Drawing for the job (mm, zero at the part's lowest x, y, z). Round coordinates to 2 decimals unless told otherwise and drop trailing zeros. Loops run counter-clockwise (first coordinate to the right, second up) from the corner with the lowest first, then second, coordinate; pieces in that order, holes last. Notation, with made-up numbers: (18.5, 84.25) -> (74.5, 84.25) arc R25 ccw to (74.5, 114.25) -> close; hole circle Ø11 at (32.25, 47). An arc over 180 degrees is marked (long way). Put each result on its own line as item: value. Start each with the question number.
Item 1: Cut at B-B, the plane x = 20. List the corners of the cut face in (y, z).
Item 2: Cut at C-C, the plane z = 2.45. List the corners of the cut face in (x, y), plus the area to 3 significant figures.
Item 3: Cut at A-A, the plane y = 12.5. List the corners of the cut face in (x, z).
Item 4: Drill centre lines: probe 1 along Y at (x, z) = (20, 2.2); probe 2 along X at (y, z) = (11.75, 0.25); probe 3 along X at (y, z) = (16.75, 2.85). Where is each one in solid material? Low to high. Write a range as [from, to].
Item 5: Pull direction X, two halves, no side cores. Call the marked faces 1 and 2: +X half, -X half, draft (parallel to the pull), parting line (faces both ways), or undercut.
Item 6: Flat gauge pin, fed straight in: pin 1 Ø10 at (x, y) = (20, 12.5) entering from -Z. Where does the tip first touch, or does it go through?
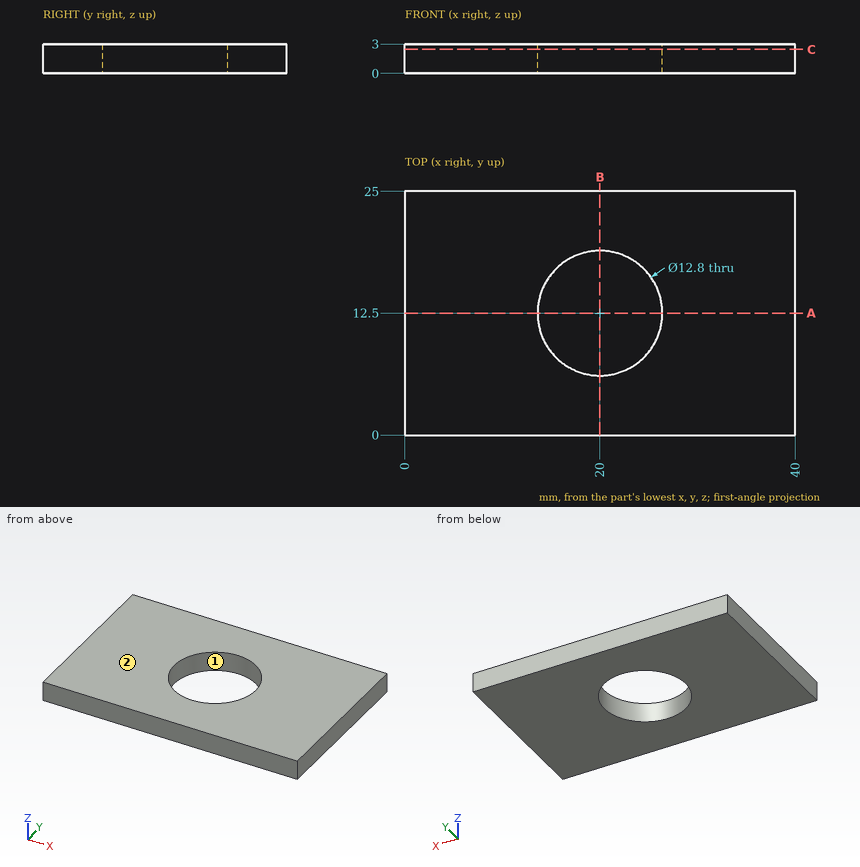
Reply:
1. outline: (0, 0) -> (6.1, 0) -> (6.1, 3) -> (0, 3) -> close; (18.9, 0) -> (25, 0) -> (25, 3) -> (18.9, 3) -> close
2. outline: (0, 0) -> (40, 0) -> (40, 25) -> (0, 25) -> close; hole circle Ø12.8 at (20, 12.5)
2. area: 871 mm^2
3. outline: (0, 0) -> (13.6, 0) -> (13.6, 3) -> (0, 3) -> close; (26.4, 0) -> (40, 0) -> (40, 3) -> (26.4, 3) -> close
4. probe 1: y = [0, 6.1], [18.9, 25]
4. probe 2: x = [0, 13.64], [26.36, 40]
4. probe 3: x = [0, 15.21], [24.79, 40]
5. face 1: undercut
5. face 2: draft
6. pin 1: passes through
